The model under review builds one solid part; all positions refer to its coordinate system, in mm. Face numbers are marked on the shaded views. A direction names the side the tool comes from. Coordinates: 2 decimals unless noted, no trailing zeros. Order: outer loops, then holes, each group sorted by start corner. A loop starts at its lowest first (then second) coordinate and runs counter-clockwise, first axis right, second up. Notation, with made-up numbers: (6.5, -28.75) -> (58.5, -28.75) arc R17 cw to (58.5, -16.75) -> close; hole circle Ø5 at (60.5, 19). An arc over 180 degrees is marked (long way). Use CSV: the item, a comma, the result in double quotes. Start each with the question number.
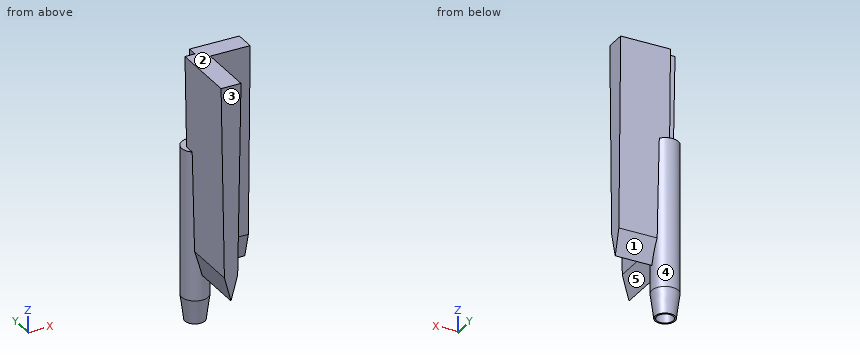
```python
from build123d import *

# Parameters (mm, degrees)
F3_DEPTH = 4
F5_DEPTH = 3


with BuildPart() as f1:
    # F0 (on Front) → F1 (revolve)
    with BuildSketch(Plane.XZ):
        Polygon((-0.25, 10.5), (-0.8, 10.5), (-0.8, 1.5), (-0.6, 0), (-0.5, 0), (-0.5, 10), align=None)
    revolve(axis=Axis((0, 0, 5.25), (0, 0, -1)))

    # F2 (on Front) → F3 (join)
    with BuildSketch(Plane.XZ):
        Polygon((0.6, 16), (-0.6, 16), (-0.4, 4.49282), (0, 3), (0.4, 4.49282), align=None)
    extrude(amount=F3_DEPTH)

    # F4 (on Right) → F5 (join)
    with BuildSketch(Plane.YZ):
        Polygon((0.6, 16), (-0.6, 16), (-0.4, 4.49282), (0, 3), (0.4, 4.49282), align=None)
    extrude(amount=F5_DEPTH)


solid = f1.part
```
Q1. Add section D-D, the plane z = 3.25. State the section outline as (x, y) points.
Q2. To check wall thickness, follow probe 1 along Y at (x, z) = (0, 2.75); probe 2 along X at (y, z) = (0.1, 11.5); probe 3 along Y at (x, z) = (-0.3, 3.5). State the ranges of each line that lie inside material, in increasing order.
Q3. Clearance check with a flat-ended pin moving along its axis: pin 1 Ø0.7 at (y, z) = (0.5, 9.5) entering from -X. State where the tip first meets the part, or that it passes through.
Q4. Add section A-A, the plane y = -3.55. State the section outline as (x, z) points.
Q5. Add section B-B, the plane z = 12.5. State the section outline as (x, y) points, then the cut area to 3 significant figures.
Q6. For the marked faces 1, 2, 3, 4 and 5, list the 3-axis set-ups (+Z, -Z, +X, -X, +Y, -Y) from which the entire face can be reached by the end or side of a thin tool; tool diameter is ignored.
Answer block:
1,outline,"(-0.07, -4) -> (0.07, -4) -> (0.07, -0.8) arc R0.8 ccw to (0.8, -0.07) -> (3, -0.07) -> (3, 0.07) -> (0.8, 0.07) arc R0.8 ccw (long way) to (-0.07, -0.8) -> close; hole (-0.07, -0.5) -> (-0.07, 0) -> (0, 0) -> (0, 0.07) -> (0.5, 0.07) arc R0.5 ccw (long way) to start; hole (0.07, -0.5) arc R0.5 ccw to (0.5, -0.07) -> (0.07, -0.07) -> close"
2,probe 1,"y = -0.8 to -0.5, 0.5 to 0.8"
2,probe 2,"x = 0 to 3"
2,probe 3,"y = -0.74 to -0.4, 0.4 to 0.74"
3,pin 1,"stops at x = -0.79"
4,outline,"(-0.6, 16) -> (-0.4, 4.49) -> (0, 3) -> (0.4, 4.49) -> (0.6, 16) -> close"
5,outline,"(-0.54, -4) -> (0.54, -4) -> (0.54, -0.54) -> (3, -0.54) -> (3, 0.54) -> (0, 0.54) -> (0, 0) -> (-0.54, 0) -> close"
5,area,"7.26 mm²"
6,face 1,"-Z, +X, +Y"
6,face 2,"+Z, +X, -X, +Y, -Y"
6,face 3,"+Z, -Z, +X, -X, -Y"
6,face 4,"-Z"
6,face 5,"-Z, +X, -Y"
